from build123d import *

# Parameters (mm, degrees)
SKETCH1_W           = 250
SKETCH1_H           = 6.75396212
BOSS_EXTRUDE2_DEPTH = 50
SKETCH2_W           = 6.75
SKETCH2_H           = 250
BOSS_EXTRUDE3_DEPTH = 50
BOSS_EXTRUDE4_DEPTH = 50
FILLET1_R           = 10
FILLET2_R           = 10
FILLET3_R           = 10
FILLET4_R           = 10
FILLET5_R           = 10
FILLET6_R           = 10
SKETCH5_W           = 6.75
SKETCH5_H           = 50
BOSS_EXTRUDE5_DEPTH = 250
FILLET7_R           = 10


with BuildPart() as part:
    # Sketch1 → Boss-Extrude2 (new body)
    with BuildSketch(Plane(origin=(0, 0, 0), x_dir=(1, 0, 0), z_dir=(0, 1, 0))):
        with Locations((-125, 3.37698106)):
            Rectangle(SKETCH1_W, SKETCH1_H)
    extrude(amount=BOSS_EXTRUDE2_DEPTH)

    # Sketch2 → Boss-Extrude3 (add)
    with BuildSketch(Plane(origin=(0, 0, 0), x_dir=(1, 0, 0), z_dir=(0, 1, 0))):
        with Locations((-246.625, 125)):
            Rectangle(SKETCH2_W, SKETCH2_H)
    extrude(amount=BOSS_EXTRUDE3_DEPTH)

    # Sketch3 → Boss-Extrude4 (add)
    with BuildSketch(Plane(origin=(0, 0, 0), x_dir=(1, 0, 0), z_dir=(0, 1, 0))):
        Polygon((-243.25, 128.37698106), (-121.625, 6.75396212), (-121.625, 0), (-250, 125), align=None)
    extrude(amount=BOSS_EXTRUDE4_DEPTH)

    # Fillet1
    fillet1_edges = [part.edges().sort_by_distance(p)[0] for p in [
        (-250, 25, 0),
    ]]
    fillet(fillet1_edges, radius=FILLET1_R)

    # Fillet2
    fillet2_edges = [part.edges().sort_by_distance(p)[0] for p in [
        (-243.25, 25, -6.75396212),
    ]]
    fillet(fillet2_edges, radius=FILLET2_R)

    # Fillet3
    fillet3_edges = [part.edges().sort_by_distance(p)[0] for p in [
        (-243.25, 25, -118.427458617),
    ]]
    fillet(fillet3_edges, radius=FILLET3_R)

    # Fillet4
    fillet4_edges = [part.edges().sort_by_distance(p)[0] for p in [
        (-128.561319097, 25, -6.75396212),
    ]]
    fillet(fillet4_edges, radius=FILLET4_R)

    # Fillet5
    fillet5_edges = [part.edges().sort_by_distance(p)[0] for p in [
        (-121.625, 25, -6.75396212),
    ]]
    fillet(fillet5_edges, radius=FILLET5_R)

    # Fillet6
    fillet6_edges = [part.edges().sort_by_distance(p)[0] for p in [
        (-243.25, 25, -128.37698106),
    ]]
    fillet(fillet6_edges, radius=FILLET6_R)

    # Sketch5 → Boss-Extrude5 (add)
    with BuildSketch(Plane(origin=(0, 0, 0), x_dir=(1, 0, 0), z_dir=(0, 1, 0))):
        with Locations((-246.625, 225)):
            Rectangle(SKETCH5_W, SKETCH5_H)
    extrude(amount=BOSS_EXTRUDE5_DEPTH)

    # Fillet7
    fillet7_edges = [part.edges().sort_by_distance(p)[0] for p in [
        (-246.625, 50, -200),
    ]]
    fillet(fillet7_edges, radius=FILLET7_R)


solid = part.part
Model file for the job. Use its own axes, mm. A direction names the side the tool comes from. Give positions to 0.01 mm unless a question says otherwise; leave off trailing zeros. Order: outer loops, then holes, each group sorted by start corner. A loop starts at its lowest first (then second) coordinate and runs counter-clockwise, first axis right, second up. Notation, with made-up numbers: (64, 47.25) - (111, 47.25) arc R21 ccw to (111, 86.25) - close; hole circle Ø1 at (31.5, 40). An arc over 180 degrees is marked (long way). One line per item, written item: value.
Item 1: Slice it at D-D (z = -160). List the corners of the cut face in (x, y), then the cut area to 4 significant figures.
Response values:
outline: (-250, 0) - (-243.25, 0) - (-243.25, 50) - (-250, 50) - close
area: 337.5 mm2
Item 2: Slice it at B-B (x = -215). List the corners of the cut face in (y, z), then the cut area to 3 significant figures.
Response values:
outline: (0, -100.13) - (50, -100.13) - (50, -90.92) - (0, -90.92) - close; (0, -6.75) - (50, -6.75) - (50, 0) - (0, 0) - close
area: 798 mm2
Item 3: Slice it at A-A (z = -72). List the corners of the cut face in (x, y).
Response values:
outline: (-250, 0) - (-243.25, 0) - (-243.25, 50) - (-250, 50) - close; (-195.57, 0) - (-186.87, 0) - (-186.87, 50) - (-195.57, 50) - close
Item 4: Tool access for faces 4 (the flat face through (-122, 25, 0)), 5 (the flat face through (-250, 68, -208)), 6 (the cylindrical face through (-237.29, 25.35, -103.88)), 7 (the flat face through (-243.25, 95, -217)), 8 (the flat face through (-180, 50, -60)): list every direction of +Z, -Z, +X, -X, +Y, -Y with a clear straight run to the whole face (end or side of a thin tool).
Response values:
face 4: +Z, +X, -X, +Y, -Y
face 5: +Z, -Z, -X, +Y, -Y
face 6: +Y, -Y
face 7: -Z, +X, +Y, -Y
face 8: +Z, +X, -X, +Y
Item 5: Slice it at C-C (x = -83.5). List the corners of the cut face in (y, z), then the cut area to 3 significant figures.
Response values:
outline: (0, -6.75) - (50, -6.75) - (50, 0) - (0, 0) - close
area: 338 mm2
Item 6: Pin check, flat tips, straight feed: pin 1 Ø25 at (x, y) = (-186.5, 31) entering from -Z; pin 2 Ø5.5 at (x, y) = (-248, 149) entering from +Z; pin 3 Ø10 at (x, z) = (-191, -83) entering from +Y. Stop position of each tip, or through.
Response values:
pin 1: z = -84.13
pin 2: z = -200
pin 3: y = 50
Item 7: Wall check: line 1 (X direction, y = 230.5, z = -215.5); line 2 (Z direction, x = -18, y = 49). Give the ranges that are in metal, low to high.
Response values:
line 1: -250 to -243.25
line 2: -6.75 to 0
Item 8: Two-plate mould, pull along X, no slides. Class faces 1 (the cylindrical face through (-240.4, 25.35, -9.76)), 2 (the cylindrical face through (-242.468, 25.35, -128.642)), 3 (the flat face through (-247, 250, -225)): released by +X, released by -X, zero draft, split by the parting line, or undercut.
Response values:
face 1: undercut
face 2: released by +X
face 3: zero draft
